Part model, mm, in its own coordinate system. Coordinates: 2 decimals unless noted, no trailing zeros. Order: outer loops, then holes, each group sorted by start corner. A loop starts at its lowest first (then second) coordinate and runs counter-clockwise, first axis right, second up.
1) Cut at D-D (x = -29). List the corners of the cut face in (y, z).
2) Wall check: L1, parallel to Y at x = -33, z = 1.9; L2, parallel to X at y = -14, z = 2.65; L3, parallel to X at y = 13, z = 2.8. Give the ranges that are in metal, low to high.
3) Cut at C-C (z = 0.65). Give the number of separate pieces and of enclosed holes in the cut face, and give its area (3 significant figures).
4) Cut at A-A (y = 0). List the corners of the cut face in (x, z).
5) Pin check, flat tips, straight feed: pin 1 Ø0.9 at (x, z) = (38, 1) entering from -Y; pin 2 Ø1.5 at (y, z) = (-10.5, 2) entering from -X; pin 3 Ø1 at (y, z) = (-57, 1) entering from +X. Stop position of each tip, or through.
6) Cut at B-B (x = 0.5). List the corners of the cut face in (y, z), and give its area (3 significant figures).
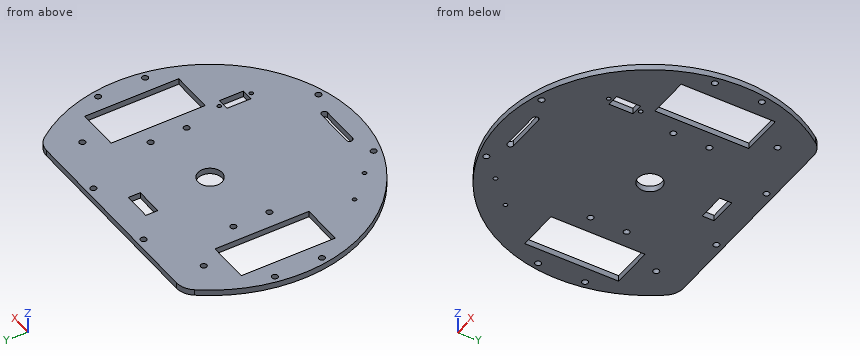
```python
from build123d import *

# Parameters (mm, degrees)
SKETCH1_R           = 1.5
SKETCH1_R_2         = 6
SKETCH1_R_3         = 1
SKETCH1_W           = 21
SKETCH1_H           = 47
SKETCH1_W_2         = 6
SKETCH1_H_2         = 12
SKETCH1_W_3         = 14
SKETCH1_H_3         = 6
BOSS_EXTRUDE2_DEPTH = 3


with BuildPart() as part:
    # Sketch1 → Boss-Extrude2 (new body)
    with BuildSketch(Plane.XY):
        with BuildLine():
            Line((-51.796300436, 49.270131922), (51.796300436, 49.270131922))
            ThreePointArc((51.796300436, 49.270131922), (56.24514368, 48.226012325), (59.764962041, 45.311690679))
            ThreePointArc((59.764962041, 45.311690679), (0, -75), (-59.764962041, 45.311690679))
            ThreePointArc((-59.764962041, 45.311690679), (-56.24514368, 48.226012325), (-51.796300436, 49.270131922))
        make_face()
        with Locations((22.094715098, -68.059231897)):
            Circle(SKETCH1_R, mode=Mode.SUBTRACT)
        with Locations((-22.094715098, -68.000540915)):
            Circle(SKETCH1_R, mode=Mode.SUBTRACT)
        Circle(SKETCH1_R_2, mode=Mode.SUBTRACT)
        with Locations((-33, 9)):
            Circle(SKETCH1_R, mode=Mode.SUBTRACT)
        with Locations((-33, -9)):
            Circle(SKETCH1_R, mode=Mode.SUBTRACT)
        with Locations((48.430328075, 33.5)):
            Circle(SKETCH1_R, mode=Mode.SUBTRACT)
        with Locations((20, 45.770131922)):
            Circle(SKETCH1_R, mode=Mode.SUBTRACT)
        with Locations((-20, 45.770131922)):
            Circle(SKETCH1_R, mode=Mode.SUBTRACT)
        with Locations((-48.430328075, 33.5)):
            Circle(SKETCH1_R, mode=Mode.SUBTRACT)
        with Locations((-32.419192278, -56.938528011)):
            Circle(SKETCH1_R_3, mode=Mode.SUBTRACT)
        with Locations((-45.012826675, -44.077720389)):
            Circle(SKETCH1_R_3, mode=Mode.SUBTRACT)
        with Locations((37.944032627, -28.385695159)):
            Circle(SKETCH1_R_3, mode=Mode.SUBTRACT)
        with Locations((37.944032627, -44.385695159)):
            Circle(SKETCH1_R_3, mode=Mode.SUBTRACT)
        with Locations((-70.527920003, 11.75)):
            Circle(SKETCH1_R, mode=Mode.SUBTRACT)
        with Locations((-70.527920003, -11.75)):
            Circle(SKETCH1_R, mode=Mode.SUBTRACT)
        with Locations((70.527920003, -11.75)):
            Circle(SKETCH1_R, mode=Mode.SUBTRACT)
        with Locations((70.527920003, 11.75)):
            Circle(SKETCH1_R, mode=Mode.SUBTRACT)
        with Locations((33, -9)):
            Circle(SKETCH1_R, mode=Mode.SUBTRACT)
        with Locations((33, 9)):
            Circle(SKETCH1_R, mode=Mode.SUBTRACT)
        with Locations((-51.930328075, 0)):
            Rectangle(SKETCH1_W, SKETCH1_H, mode=Mode.SUBTRACT)
        with BuildLine():
            Line((-10, -62), (10, -62))
            ThreePointArc((10, -62), (11.5, -63.5), (10, -65))
            Line((10, -65), (-10, -65))
            ThreePointArc((-10, -65), (-11.5, -63.5), (-10, -62))
        make_face(mode=Mode.SUBTRACT)
        with Locations((37.944032627, -36.385695159)):
            Rectangle(SKETCH1_W_2, SKETCH1_H_2, mode=Mode.SUBTRACT)
        with Locations((51.930328075, 0)):
            Rectangle(SKETCH1_W, SKETCH1_H, mode=Mode.SUBTRACT)
        with Locations((0, 33.5)):
            Rectangle(SKETCH1_W_3, SKETCH1_H_3, mode=Mode.SUBTRACT)
    extrude(amount=BOSS_EXTRUDE2_DEPTH)


solid = part.part
```
Geometry check:
1. outline: (-69.17, 0) - (49.27, 0) - (49.27, 3) - (-69.17, 3) - close
2. L1: y = -67.35 to -57.75, -56.12 to -10.5, -7.5 to 7.5, 10.5 to 49.27
2. L2: x = -73.68 to -62.43, -41.43 to 41.43, 62.43 to 73.68
2. L3: x = -73.86 to -71.36, -69.7 to -62.43, -41.43 to 41.43, 62.43 to 69.7, 71.36 to 73.86
3. separate pieces: 1
3. enclosed holes: 24
3. area: 13,200 mm2
4. outline: (-75, 0) - (-62.43, 0) - (-62.43, 3) - (-75, 3) - close; (-41.43, 0) - (-6, 0) - (-6, 3) - (-41.43, 3) - close; (6, 0) - (41.43, 0) - (41.43, 3) - (6, 3) - close; (62.43, 0) - (75, 0) - (75, 3) - (62.43, 3) - close
5. pin 1: stops at y = -64.92
5. pin 2: stops at x = -74.36
5. pin 3: stops at x = 49.32
6. outline: (-75, 0) - (-65, 0) - (-65, 3) - (-75, 3) - close; (-62, 0) - (-5.98, 0) - (-5.98, 3) - (-62, 3) - close; (5.98, 0) - (30.5, 0) - (30.5, 3) - (5.98, 3) - close; (36.5, 0) - (49.27, 0) - (49.27, 3) - (36.5, 3) - close
6. area: 310 mm2
